Can you work these out from the model? Positions are in its coordinate system, mm. A direction names the side the tool comes from. Give positions to 0.01 mm unless a question says otherwise; leave off trailing zeros. Loops run counter-clockwise (first coordinate to the right, second up) from the corner with the lowest first, then second, coordinate; pieces in that order, holes last. Notation, with made-up numbers: M -1.75,85.25 L 5.25,85.25 A17 ccw 5.25,89.25 Z; hole C 7.5,74 d1. An arc over 180 degrees is marked long. Answer as a JSON object with one key per item and string values.
```python
from build123d import *

# Parameters (mm, degrees)
F0_W      = 200.025
F0_H      = 76.2
F1_DEPTH  = 36.83
F2_DEPTH  = 31.75
F4_D      = 10.71626
F4_DEPTH  = 15.875
F4_TIP    = 3.2194893086
F5_D      = 12.7
F5_DEPTH  = 12.7
F5_TIP    = 3.8154649308
F6_SIZE   = 1.27
F7_R      = 9.525
F8_DEPTH  = 9.525
F10_D     = 10.71626
F10_DEPTH = 12.7
F10_TIP   = 3.2194893086


# Not quite as in the source:
# - a length typed as a fraction of an inch, garbled in the dataset ("3 / 203.2 mm" for 3/8 in), is restored
# - a feature names something its author has since deleted; it is built from what else it names


with BuildPart() as f1:
    # F0 (on Top) → F1 (new body)
    with BuildSketch(Plane.XY):
        with Locations((-0.1895949244, 0.1812406208)):
            Rectangle(F0_W, F0_H)
    extrude(amount=F1_DEPTH)

    # F2 (cut): a face of the model
    f2_faces = [f1.faces().sort_by_distance(p)[0] for p in [
        (-0.1895949244, 38.2812406208, 18.415),
    ]]
    extrude(f2_faces, amount=-F2_DEPTH, mode=Mode.SUBTRACT)

    # F4
    with Locations(Plane(origin=(0, 6.5312406208, 0), x_dir=(-1, 0, 0), z_dir=(0, 1, 0))):
        with Locations((-80.7729050756, 20.6248), (81.1520949244, 20.6248)):
            Hole(F4_D / 2, depth=F4_DEPTH)
            with Locations((0, 0, -(F4_DEPTH + F4_TIP / 2))):  # 118° drill point
                Cone(0, F4_D / 2, F4_TIP, mode=Mode.SUBTRACT)

    # F5
    with Locations(Plane(origin=(0, 6.5312406208, 0), x_dir=(-1, 0, 0), z_dir=(0, 1, 0))):
        with Locations((-49.0229050756, 20.6248), (49.4020949244, 20.6248)):
            Hole(F5_D / 2, depth=F5_DEPTH)
            with Locations((0, 0, -(F5_DEPTH + F5_TIP / 2))):  # 118° drill point
                Cone(0, F5_D / 2, F5_TIP, mode=Mode.SUBTRACT)

    # F6
    f6_edges = [f1.edges().sort_by_distance(p)[0] for p in [
        (-100.202095, -15.693759, 0),
        (99.822905, -15.693759, 0),
    ]]
    chamfer(f6_edges, length=F6_SIZE)

    # F7 (on face) → F8 (cut)
    with BuildSketch(Plane.XZ.offset(37.9187593792)):
        with Locations((49.0229050756, 20.6248)):
            Circle(F7_R)
    extrude(amount=-F8_DEPTH, mode=Mode.SUBTRACT)

    # F10
    with Locations(Plane.XZ.offset(28.3937593792)):
        with Locations((49.0229050756, 20.6248)):
            Hole(F10_D / 2, depth=F10_DEPTH)
            with Locations((0, 0, -(F10_DEPTH + F10_TIP / 2))):  # 118° drill point
                Cone(0, F10_D / 2, F10_TIP, mode=Mode.SUBTRACT)


solid = f1.part
```
1) For faces 1 (the cylindrical face through (53.3, -22, 17.4)), 2 (the flat face through (-2, 6.531, 18)), 3 (the cylindrical face through (43.984, 0.092, 16.761)), which set-ups out of +Z, -Z, +X, -X, +Y, -Y let a thin tool reach every point of the face, with its end or its side?
Answer list:
{"face 1": "-Y", "face 2": "+Z, -Z, +X, -X, +Y", "face 3": "+Y"}
2) If we mould it in two halves opening along X, with no side actions, what happens to faces 4 (the flat face through (99.823, -16, 19)), 5 (the flat face through (-2, -37.919, 18)), 6 (the conical face through (49.9, -9.32, 19.95)), 7 (the flat face through (53.1, -28.394, 16.5))? For each: +X half, -X half, draft (parallel to the pull), parting line (faces both ways), or undercut.
Answer list:
{"face 4": "+X half", "face 5": "draft", "face 6": "undercut", "face 7": "undercut"}
3) Suppose I cut it at A-A, the plane y = 3. Write out the boundary of the cut face in (x, z).
Answer list:
{"outline": "M -100.2,1.27 L -98.93,0 L 98.55,0 L 99.82,1.27 L 99.82,36.83 L -100.2,36.83 Z; hole C -81.15,20.62 d10.72; hole C -49.4,20.62 d12.7; hole C 49.02,20.62 d12.7; hole C 80.77,20.62 d10.72"}
4) Please list where these lines run through material, in increasing order: line 1 along Z through (x, y) = (81, -1); line 2 along X through (y, z) = (-32.5, 16); line 3 along X through (y, z) = (-32, 14). Write a range as from..to.
Answer list:
{"line 1": "0..15.27, 25.98..36.83", "line 2": "-100.2..40.7, 57.35..99.82", "line 3": "-100.2..42.18, 55.87..99.82"}
5) Will these pins go through, and if not, where does the flat tip stop? pin 1 Ø5.5 at (x, z) = (52, 16.5) entering from -Y; pin 2 Ø8.5 at (x, z) = (-81.15, 20.62) entering from +Y; pin 3 Ø10 at (x, z) = (49.02, 20.62) entering from +Y.
Answer list:
{"pin 1": "y = -28.39", "pin 2": "y = -10.01", "pin 3": "y = -6.98"}
